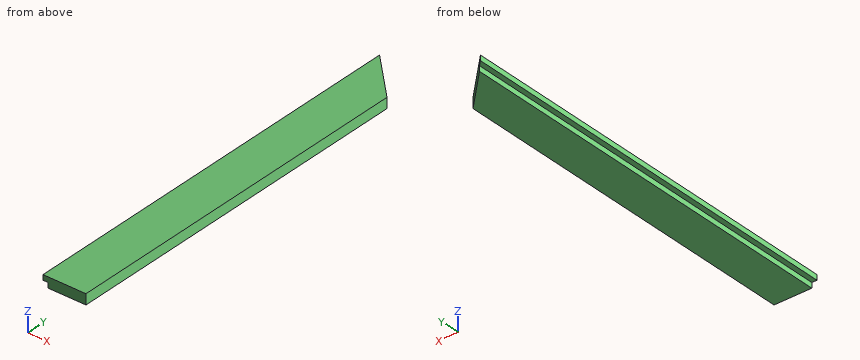
from build123d import *

# Parameters (mm, degrees)
F0_W     = 50
F0_H     = 474
F1_DEPTH = 12
F2_W     = 6
F2_H     = 474
F3_DEPTH = 6
F5_DEPTH = 12


with BuildPart() as f1:
    # F0 (on Top) → F1 (new body)
    with BuildSketch(Plane.XY):
        Rectangle(F0_W, F0_H)
    extrude(amount=F1_DEPTH)

    # F2 (on face) → F3 (cut)
    with BuildSketch(Plane(origin=(0, 0, 0), x_dir=(1, 0, 0), z_dir=(0, 0, -1))):
        with Locations((-22, 0)):
            Rectangle(F2_W, F2_H)
    extrude(amount=-F3_DEPTH, mode=Mode.SUBTRACT)

    # F4 (on face) → F5 (cut, through all)
    with BuildSketch(Plane.XY.offset(12)):
        Polygon((25, 237), (-25, 237), (25, 187), align=None)
    extrude(amount=-F5_DEPTH, mode=Mode.SUBTRACT)


solid = f1.part
The listing builds one solid part. Answer for the finished solid, in the listing's coordinates (mm). Round coordinates to 2 decimals unless told otherwise and drop trailing zeros. Order: outer loops, then holes, each group sorted by start corner. A loop starts at its lowest first (then second) coordinate and runs counter-clockwise, first axis right, second up. Notation, with made-up numbers: (34.25, 48.25) -> (89.25, 48.25) arc R20 ccw to (89.25, 73.25) -> close; hole circle Ø7 at (-21, 35.25). An arc over 180 degrees is marked (long way). Write each question's results on one line, items separated by ' | '. Start each with the question number.
Q1. Find section C-C (z = 9). Determine the outline of the cut face in (x, y).
Q2. Find section D-D (y = -203). Determine the outline of the cut face in (x, z), then the cut area to 3 significant figures.
Q3. Each of these flat-tipped pins is pushed along its axis until it touches: pin 1 (5 mm diameter, centred on y = 62, z = 2.5, fed in from -X); pin 2 (1 mm diameter, centred on x = 14.5, z = 4, fed in from +Y); pin 3 (3 mm diameter, centred on x = -23, y = -77, fed in from -Z). Where does it stop, or does it pass through?
Q4. Straight lines are drawn through the part: probe 1 along X at (y, z) = (-40, 3); probe 2 along Y at (x, z) = (-8, 10.5); probe 3 along Y at (x, z) = (-12.5, 5.75). For each, find the intervals that lie inside material, in ascending order. Write a range as from..to.
Q5. Find section A-A (y = 201.5). Determine the outline of the cut face in (x, z), then the cut area to 3 significant figures.
Q6. Find section B-B (x = 11). Determine the outline of the cut face in (y, z), then the cut area to 3 significant figures.
Worked answers:
1) outline: (-25, -237) -> (25, -237) -> (25, 187) -> (-25, 237) -> close
2) outline: (-25, 6) -> (-19, 6) -> (-19, 0) -> (25, 0) -> (25, 12) -> (-25, 12) -> close | area: 564 mm2
3) pin 1: stops at x = -19 | pin 2: stops at y = 198 | pin 3: stops at z = 6
4) probe 1: x = -19..25 | probe 2: y = -237..220 | probe 3: y = -237..224.5
5) outline: (-25, 6) -> (-19, 6) -> (-19, 0) -> (10.5, 0) -> (10.5, 12) -> (-25, 12) -> close | area: 390 mm2
6) outline: (-237, 0) -> (201, 0) -> (201, 12) -> (-237, 12) -> close | area: 5,260 mm2
